from build123d import *

# Parameters (mm, degrees)
SKETCH1_R           = 1.5
BOSS_EXTRUDE1_DEPTH = 16
SKETCH2_R           = 2.6
BOSS_EXTRUDE2_DEPTH = 1.7
BOSS_EXTRUDE2_TAPER = 32
SKETCH3_W           = 0.5
SKETCH3_H           = 1.758378485
SKETCH3_H_2         = 1.741621515
SKETCH3_W_2         = 1.734727157
SKETCH3_H_3         = 0.5
SKETCH3_W_3         = 1.765272843
CUT_EXTRUDE1_DEPTH  = 0.3


with BuildPart() as part:
    # Sketch1 → Boss-Extrude1 (new body)
    with BuildSketch(Plane(origin=(0, 0, 0), x_dir=(1, 0, 0), z_dir=(0, 1, 0))):
        Circle(SKETCH1_R)
    extrude(amount=BOSS_EXTRUDE1_DEPTH)

    # Sketch2 → Boss-Extrude2 (add)
    with BuildSketch(Plane(origin=(0, 16, 0), x_dir=(1, 0, 0), z_dir=(0, 1, 0))):
        Circle(SKETCH2_R)
    extrude(amount=-BOSS_EXTRUDE2_DEPTH, taper=BOSS_EXTRUDE2_TAPER)

    # Sketch3 → Cut-Extrude1 (cut)
    with BuildSketch(Plane(origin=(0, 16, 0), x_dir=(1, 0, 0), z_dir=(0, 1, 0))):
        with Locations((-0.015272843, 1.120810757)):
            Rectangle(SKETCH3_W, SKETCH3_H)
        with Locations((-0.015272843, -1.129189243)):
            Rectangle(SKETCH3_W, SKETCH3_H_2)
        with Locations((-1.132636421, -0.008378485)):
            Rectangle(SKETCH3_W_2, SKETCH3_H_3)
        with Locations((1.117363579, -0.008378485)):
            Rectangle(SKETCH3_W_3, SKETCH3_H_3)
        with Locations((-0.015272843, -0.008378485)):
            Rectangle(SKETCH3_W, SKETCH3_H_3)
    extrude(amount=-CUT_EXTRUDE1_DEPTH, mode=Mode.SUBTRACT)


solid = part.part
Geometry: final body of the model. Coordinates: model frame, mm. Coordinates: 2 decimals unless noted, no trailing zeros. Order: outer loops, then holes, each group sorted by start corner. A loop starts at its lowest first (then second) coordinate and runs counter-clockwise, first axis right, second up. Notation, with made-up numbers: M 62.25,84.5 L 121.25,84.5 A30 cw 121.25,115.5 Z; hole C -32.75,32.5 d6. An arc over 180 degrees is marked long. One line per question, with ' | ' between items. Start each with the question number.
Item 1: Pin query (flat end, axial travel): pin 1 Ø1 at (y, z) = (3.5, 1) entering from -X; pin 2 Ø1 at (x, y) = (-1, 6.5) entering from -Z; pin 3 Ø3 at (y, z) = (3.5, -1) entering from +X. Return the tip coordinate at first contact, or that it passes through.
Item 2: Ray query, probe 1 along Y at (x, z) = (0.05, -0.5); probe 2 along X at (y, z) = (10.75, 0.1); probe 3 along Y at (x, z) = (-2, -0.7). Return the intervals inside material, ascending. Write a range as [from, to].
Item 3: Cut plane C-C, the plane y = 15. Return the cut outline in (x, z), then the cut area to 3 significant figures.
Item 4: Cut plane B-B, the plane y = 2.25. Return the cut outline in (x, z).
Item 5: Draft query along Z for faces 1 (the flat face through (0, 15.7, 0)), 2 (the flat face through (1, 16, 1)), 3 (the cylindrical face through (-1.5, 7.05, -0.07)). Return one class per face: released by +Z, released by -Z, zero draft, split by the parting line, or undercut.
A:
1) pin 1: stops at x = -1.41 | pin 2: stops at z = -1.41 | pin 3: stops at x = 1.5
2) probe 1: y = [0, 15.7] | probe 2: x = [-1.5, 1.5] | probe 3: y = [15.23, 16]
3) outline: C 0,0 d3.95 | area: 12.3 mm2
4) outline: C 0,0 d3
5) face 1: undercut | face 2: zero draft | face 3: split by the parting line
